Could you check a few things on this drawing? It's one solid part, dimensions in mm from its lowest x, y, z. A direction names the side the tool comes from. Give positions to 0.01 mm unless a question says otherwise; leave off trailing zeros. Loops run counter-clockwise (first coordinate to the right, second up) from the corner with the lowest first, then second, coordinate; pieces in that order, holes last. Notation, with made-up numbers: (-23.75, 19) - (-13.75, 19) arc R20 ccw to (-13.75, 51) - close; hole circle Ø8 at (-16.5, 11). An arc over 180 degrees is marked (long way). Write item = value, one per line.
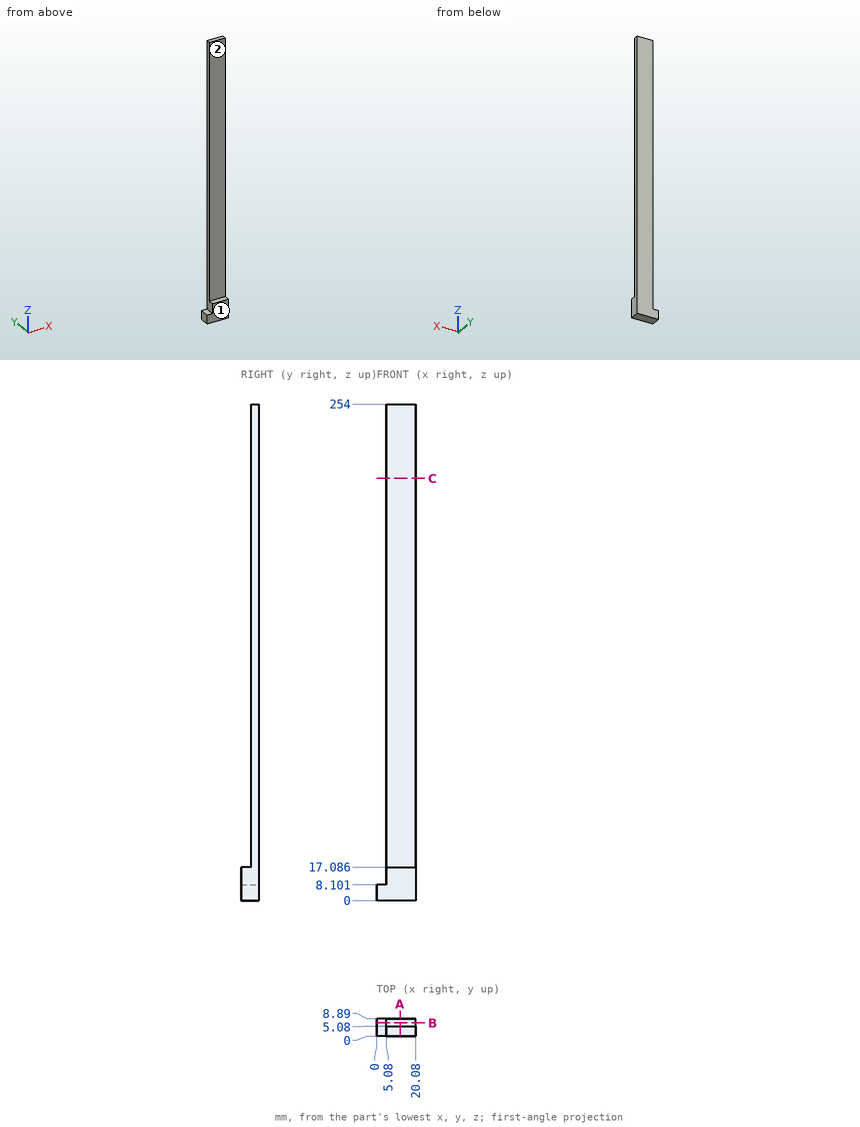
Q1. Imagine slicing it at A-A, the plane x = 12. Write out the boundary of the cut face in (y, z).
Output:
outline = (0, 0) - (8.89, 0) - (8.89, 254) - (5.08, 254) - (5.08, 17.09) - (0, 17.09) - close
Q2. Imagine slicing it at C-C, the plane z = 216. Write out the boundary of the cut face in (x, y).
Output:
outline = (5.08, 5.08) - (20.08, 5.08) - (20.08, 8.89) - (5.08, 8.89) - close
Q3. I need wall thicknesses on L1, parallel to Y at x = 10.25, z = 48; L2, parallel to Z at x = 14.5, y = 3.5; L3, parallel to X at y = 8, z = 211.5. Which ranges of each line are inside material? Lowest first, please.
Output:
L1 = 5.08 to 8.89
L2 = 0 to 17.09
L3 = 5.08 to 20.08
Q4. Which directions (+Z, -Z, +X, -X, +Y, -Y) give clear straight access to the entire face, cutting with the end or side of a thin tool? Please do the marked faces 1 and 2.
Output:
face_1 = +Z, -Z, +X, -X, -Y
face_2 = +Z, +X, -X, -Y
Q5. Imagine slicing it at B-B, the plane y = 6.75. Write out the boundary of the cut face in (x, z), then the cut area to 3 significant figures.
Output:
outline = (0, 0) - (20.08, 0) - (20.08, 254) - (5.08, 254) - (5.08, 8.1) - (0, 8.1) - close
area = 3,850 mm2
Q6. For pin 1 (5 mm diameter, centred on y = 3, z = 167.5, fed in from +X); pin 2 (3 mm diameter, centred on x = 13, y = 2, fed in from +Z); pin 3 (10 mm diameter, centred on x = 6, z = 218.5, fed in from -Y), each with a flat end and sliding along its axis, tell me the tip position at first contact or that it passes through.
Output:
pin_1 = 20.08
pin_2 = 17.09
pin_3 = 5.08
